Autodesk Inventor part; units mm, degrees
ref_plane "YZ Plane" through (0, 0, 0) normal (1, 0, 0) x (0, 1, 0)
ref_plane "XZ Plane" through (0, 0, 0) normal (0, 1, 0) x (-1, 0, 0)
ref_plane "XY Plane" through (0, 0, 0) normal (0, 0, 1) x (1, 0, 0)
sketch "Sketch1" plane through (0, 0, 0) normal (0, 0, 1) x (1, 0, 0)
  line L0 (-103, 11) -> (0, 11)
  line L1 (0, 11) -> (0, 12)
  line L2 (-1, 13) -> (-80, 13)
  line L3 (-80, 13) -> (-80, 20)
  line L4 (-80, 20) -> (-88, 20)
  line L5 (-103, 13) -> (-103, 11)
  line L6 (-103, 13) -> (-103, 15.5)
  line L7 (-102, 16.5) -> (-88, 16.5)
  line L8 (-88, 20) -> (-88, 16.5)
  line L9 (0, 12) -> (-1, 13)
  line L10 (-102, 16.5) -> (-103, 15.5)
  line L11 (-118.5, 0) -> (44.527, 0) construction
  point P0 (0, 0)
  point P1 (0, 13)
  point P2 (-84, 20)
  point P3 (-103, 16.5)
  dimension "d0" = 103
  dimension "d1" = 11
  dimension "d2" = 0
  dimension "d4" = 8
  dimension "d5" = 80
  dimension "d7" = 13
  dimension "d11" = 15
  dimension "d12" = 16.5
  dimension "d13" = 20
  dimension "d14" = 1
  dimension "d15" = 1
  dimension "d16" = 1
  dimension "d17" = 1
revolve "Revolution1" add sketch "Sketch1" angle 360 about axis through (-118.5, 0, 0) along (1, 0, 0)
properties part number "Bucha do Ferramental"
The listing builds one solid part. Answer for the finished solid, in the listing's coordinates (mm). A direction names the side the tool comes from. Give positions to 0.01 mm unless a question says otherwise; leave off trailing zeros. Order: outer loops, then holes, each group sorted by start corner. A loop starts at its lowest first (then second) coordinate and runs counter-clockwise, first axis right, second up. Notation, with made-up numbers: (12.25, 14.25) - (39.25, 14.25) arc R17 cw to (39.25, 18.25) - close; hole circle Ø7 at (41, 21). An arc over 180 degrees is marked (long way). Answer in a Markdown table with one row per item. Add a question column.
Q1. The part is cut by section A-A (y = 0). Determine the outline of the cut face in (x, z), then the cut area to 3 significant figures.
Q2. For a pull along Y with two mould halves and no side action, classify faces 1 (the cylindrical face through (-50.78, -2.38, -10.74)), 2 (the cylindrical face through (-41.053, -10.316, 7.91)), 3 (the flat face through (-88, 2.9, 16.4)) as released by +Y, released by -Y, zero draft, split by the parting line, or undercut.
Q3. Given P1, Ø20, axis at y = 7, z = -1, coming from the +X side; P2, Ø1, axis at y = -5, z = 15.5, coming from the -X side; P3, Ø6, axis at x = -33.5, y = -2, coming from the -Z side; P4, Ø12, axis at x = -29, y = -9, coming from the +Z side, each flat-ended and moving along its own axis, determine where each tip first touches the part or whether it passes through.
Q4. Which of the six approach directions +Z, -Z, +X, -X, +Y, -Y give full straight-line access (tool end or side, diameter ignored) to faces 4 (the cylindrical face through (-94.9, 15.24, -6.32)), 5 (the cylindrical face through (-84.056, -4.336, 19.524)), 6 (the flat face through (-80, 13, -4))?
Q5. The part is cut by section C-C (x = -86). Determine the outline of the cut face in (y, z), then the cut area to 3 significant figures.
Q6. The part is cut by section D-D (x = -14.5). Determine the outline of the cut face in (y, z), then the cut area to 3 significant figures.
Q7. Find the intervals of material crossed by line 1 along Y through (x, z) = (-62.5, 0.5); line 2 along Z through (x, y) = (-68, 0); line 3 along Z through (x, y) = (-81, 0), in increasing order. Write a range as [from, to].
Determined:
| question | item | result |
|---|---|---|
| 1 | outline | (-103, -15.5) - (-102, -16.5) - (-88, -16.5) - (-88, -20) - (-80, -20) - (-80, -13) - (-1, -13) - (0, -12) - (0, -11) - (-103, -11) - close; (-103, 11) - (0, 11) - (0, 12) - (-1, 13) - (-80, 13) - (-80, 20) - (-88, 20) - (-88, 16.5) - (-102, 16.5) - (-103, 15.5) - close |
| 1 | area | 627 mm² |
| 2 | face 1 | undercut |
| 2 | face 2 | split by the parting line |
| 2 | face 3 | zero draft |
| 3 | P1 | stops at x = 0 |
| 3 | P2 | stops at x = -102.71 |
| 3 | P3 | stops at z = -13 |
| 3 | P4 | stops at z = 12.65 |
| 4 | face 4 | -X |
| 4 | face 5 | +X, -X |
| 4 | face 6 | +X |
| 5 | outline | circle Ø40 at (0, 0); hole circle Ø22 at (0, 0) |
| 5 | area | 877 mm² |
| 6 | outline | circle Ø26 at (0, 0); hole circle Ø22 at (0, 0) |
| 6 | area | 151 mm² |
| 7 | line 1 | y = [-12.99, -10.99], [10.99, 12.99] |
| 7 | line 2 | z = [-13, -11], [11, 13] |
| 7 | line 3 | z = [-20, -11], [11, 20] |
